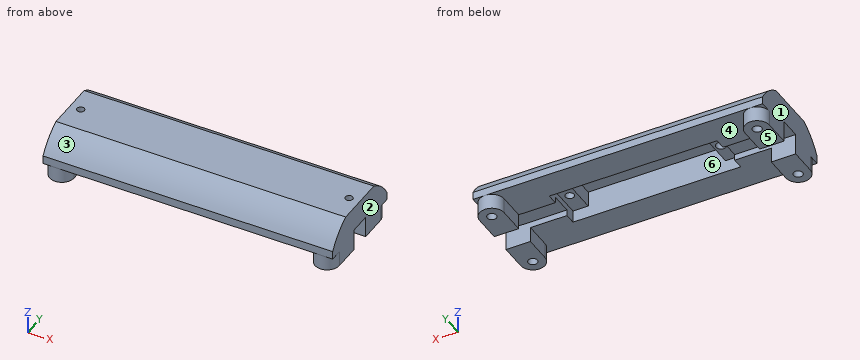
from build123d import *

# Parameters (mm, degrees)
SKETCH1_R             = 4
SKETCH1_R_2           = 1.5
BOSS_EXTRUDE1_DEPTH   = 5
BOSS_EXTRUDE1_2_DEPTH = 5
BOSS_EXTRUDE1_3_DEPTH = 5
BOSS_EXTRUDE1_4_DEPTH = 5
SKETCH2_W             = 95
SKETCH2_H             = 32.5
BOSS_EXTRUDE2_DEPTH   = 10
SKETCH3_W             = 45
SKETCH3_H             = 14.2
CUT_EXTRUDE1_DEPTH    = 9
SKETCH4_W             = 5
SKETCH4_H             = 14.2
SKETCH4_W_2           = 45
CUT_EXTRUDE2_DEPTH    = 4
SKETCH5_R             = 1.4
SKETCH5_R_2           = 1.6
CUT_EXTRUDE3_DEPTH    = 5
BOSS_EXTRUDE3_DEPTH   = 5
CUT_EXTRUDE5_DEPTH    = 96
SKETCH9_W             = 7
SKETCH9_H             = 7
CUT_EXTRUDE6_DEPTH    = 96
SKETCH10_R            = 1.2
CUT_EXTRUDE7_DEPTH    = 16


with BuildPart() as part:
    # Sketch1 → Boss-Extrude1 (new body)
    with BuildSketch(Plane.XY):
        with Locations((-43.5, -12.25)):
            Circle(SKETCH1_R)
        with Locations((-43.5, -12.25)):
            Circle(SKETCH1_R_2, mode=Mode.SUBTRACT)
    extrude(amount=BOSS_EXTRUDE1_DEPTH)



with BuildPart() as body_2:
    # Sketch1 → Boss-Extrude1 2 (new body)
    with BuildSketch(Plane.XY):
        with Locations((-43.5, 12.25)):
            Circle(SKETCH1_R)
        with Locations((-43.5, 12.25)):
            Circle(SKETCH1_R_2, mode=Mode.SUBTRACT)
    extrude(amount=BOSS_EXTRUDE1_2_DEPTH)


with BuildPart() as body_3:
    # Sketch1 → Boss-Extrude1 3 (new body)
    with BuildSketch(Plane.XY):
        with Locations((43.5, -12.25)):
            Circle(SKETCH1_R)
        with Locations((43.5, -12.25)):
            Circle(SKETCH1_R_2, mode=Mode.SUBTRACT)
    extrude(amount=BOSS_EXTRUDE1_3_DEPTH)


with BuildPart() as body_4:
    # Sketch1 → Boss-Extrude1 4 (new body)
    with BuildSketch(Plane.XY):
        with Locations((43.5, 12.25)):
            Circle(SKETCH1_R)
        with Locations((43.5, 12.25)):
            Circle(SKETCH1_R_2, mode=Mode.SUBTRACT)
    extrude(amount=BOSS_EXTRUDE1_4_DEPTH)


with BuildPart() as part_1:
    add(part.part)

    add(body_2.part)  # Boss-Extrude2 merges body 2

    add(body_3.part)  # Boss-Extrude2 merges body 3

    add(body_4.part)  # Boss-Extrude2 merges body 4
    # Sketch2 → Boss-Extrude2 (add)
    with BuildSketch(Plane.XY.offset(5)):
        Rectangle(SKETCH2_W, SKETCH2_H)
    extrude(amount=BOSS_EXTRUDE2_DEPTH)

    # Sketch3 → Cut-Extrude1 (cut)
    with BuildSketch(Plane(origin=(0, 0, 5), x_dir=(-1, 0, 0), z_dir=(0, 0, -1))):
        Rectangle(SKETCH3_W, SKETCH3_H)
    extrude(amount=-CUT_EXTRUDE1_DEPTH, mode=Mode.SUBTRACT)

    # Sketch4 → Cut-Extrude2 (cut)
    with BuildSketch(Plane(origin=(0, 0, 5), x_dir=(-1, 0, 0), z_dir=(0, 0, -1))):
        with Locations((-25, 0)):
            Rectangle(SKETCH4_W, SKETCH4_H)
        Rectangle(SKETCH4_W_2, SKETCH4_H)
        with Locations((25, 0)):
            Rectangle(SKETCH4_W, SKETCH4_H)
    extrude(amount=-CUT_EXTRUDE2_DEPTH, mode=Mode.SUBTRACT)

    # Sketch5 → Cut-Extrude3 (cut)
    with BuildSketch(Plane(origin=(0, 0, 9), x_dir=(-1, 0, 0), z_dir=(0, 0, -1))):
        with Locations((-24.8, -0.2)):
            Circle(SKETCH5_R)
        with Locations((24.8, -0.2)):
            Circle(SKETCH5_R_2)
    extrude(amount=-CUT_EXTRUDE3_DEPTH, mode=Mode.SUBTRACT)

    # Sketch6 → Boss-Extrude3 (add)
    with BuildSketch(Plane(origin=(0, 0, 5), x_dir=(-1, 0, 0), z_dir=(0, 0, -1))):
        with BuildLine():
            ThreePointArc((47.5, 12.25), (43.5, 8.25), (39.5, 12.25))
            Line((39.5, 12.25), (39.5, -12.25))
            ThreePointArc((39.5, -12.25), (43.5, -8.25), (47.5, -12.25))
            Line((47.5, -12.25), (47.5, 12.25))
        make_face()
        with BuildLine():
            ThreePointArc((-39.5, 12.25), (-43.5, 8.25), (-47.5, 12.25))
            Line((-47.5, 12.25), (-47.5, -12.25))
            ThreePointArc((-47.5, -12.25), (-43.5, -8.25), (-39.5, -12.25))
            Line((-39.5, -12.25), (-39.5, 12.25))
        make_face()
    extrude(amount=BOSS_EXTRUDE3_DEPTH)

    # Sketch8 → Cut-Extrude5 (cut, through all)
    with BuildSketch(Plane(origin=(47.5, 0, 0), x_dir=(0, 0, -1), z_dir=(1, 0, 0))):
        with BuildLine():
            ThreePointArc((-15, 8.377014021), (-11.841659381, 12.867099577), (-7.518238456, 16.25))
            Line((-7.518238456, 16.25), (-15, 16.25))
            Line((-15, 16.25), (-15, 8.377014021))
        make_face()
        with BuildLine():
            Line((-15, -16.25), (-7.688934819, -16.25))
            ThreePointArc((-7.688934819, -16.25), (-11.909309532, -12.893789895), (-15, -8.475267356))
            Line((-15, -8.475267356), (-15, -16.25))
        make_face()
    extrude(amount=-CUT_EXTRUDE5_DEPTH, mode=Mode.SUBTRACT)

    # Sketch9 → Cut-Extrude6 (cut, through all)
    with BuildSketch(Plane.ZY.offset(47.5)):
        with Locations((3.5, 0)):
            Rectangle(SKETCH9_W, SKETCH9_H)
    extrude(amount=-CUT_EXTRUDE6_DEPTH, mode=Mode.SUBTRACT)

    # Sketch10 → Cut-Extrude7 (cut, through all)
    with BuildSketch(Plane.XY.offset(15)):
        with Locations((-44, -0.049126667)):
            Circle(SKETCH10_R)
        with Locations((44, -0.049126667)):
            Circle(SKETCH10_R)
    extrude(amount=-CUT_EXTRUDE7_DEPTH, mode=Mode.SUBTRACT)


solid = part_1.part
Can you work these out from the model? Positions are in its coordinate system, mm. Face numbers are marked on the shaded views. A direction names the side the tool comes from. Coordinates: 2 decimals unless noted, no trailing zeros. Order: outer loops, then holes, each group sorted by start corner. A loop starts at its lowest first (then second) coordinate and runs counter-clockwise, first axis right, second up. Notation, with made-up numbers: M -26.5,5 L -2.5,5 A25 cw -2.5,28 Z; hole C 60,84 d11. An arc over 180 degrees is marked long. Write item = value, one per line.
(1) Suppose I cut it at A-A on z = 10.75. Please give me the cut outline in (x, y).
Results are:
outline = M -47.5,-14.02 L 47.5,-14.02 L 47.5,13.93 L -47.5,13.93 Z; hole C -44,-0.05 d2.4; hole C -24.8,-0.2 d3.2; hole M -22.5,-7.1 L 22.5,-7.1 L 22.5,7.1 L -22.5,7.1 Z; hole C 24.8,-0.2 d2.8; hole C 44,-0.05 d2.4
(2) I need wall thicknesses on line 1 along Y through (x, z) = (43.5, 1.6); line 2 along X through (y, z) = (0.5, 11.5); line 3 along X through (y, z) = (6, 7). Which ranges of each line are inside material? Lowest first, please. Write a range as [from, to].
Results are:
line_1 = [-16.25, -13.75], [-10.75, -3.5], [3.5, 10.75], [13.75, 16.25]
line_2 = [-47.5, -45.07], [-42.93, -26.24], [-23.36, -22.5], [22.5, 23.59], [26.01, 42.93], [45.07, 47.5]
line_3 = [-47.5, -27.5], [27.5, 47.5]
(3) Suppose I cut it at C-C on x = -11. Please give me the cut outline in (y, z), plus the area to 3 significant figures.
Results are:
outline = M -16.25,5 L -7.1,5 L -7.1,14 L 7.1,14 L 7.1,5 L 16.25,5 L 16.25,7.52 A18.75 ccw 8.38,15 L -8.48,15 A18.75 ccw -16.25,7.69 Z
area = 151 mm2
(4) If we mould it in two halves opening along X, with no side actions, what happens to the marked faces 1, 2, 3 and 4? For each: pulls with the +X half, pulls with the -X half, needs draft (parallel to the pull), parting line crosses it, or undercut.
Results are:
face_1 = pulls with the -X half
face_2 = pulls with the +X half
face_3 = needs draft
face_4 = undercut
(5) For pin 1 Ø4 at (x, y) = (-12.5, -0.5) entering from -Z; pin 2 Ø5 at (x, y) = (-43.5, 12.25) entering from +Z; pin 3 Ø10 at (x, y) = (7.5, -10) entering from -Z; pin 4 Ø2 at (x, z) = (-36.5, 3) entering from +Y, each with a flat end and sliding along its axis, tell me the tip position at first contact or that it passes through.
Results are:
pin_1 = 14
pin_2 = 14.24
pin_3 = 5
pin_4 = through
(6) Suppose I cut it at D-D on x = -24.8. Please give me the cut outline in (y, z).
Results are:
outline = M -16.25,5 L -7.1,5 L -7.1,9 L -1.8,9 L -1.8,14 L 1.4,14 L 1.4,9 L 7.1,9 L 7.1,5 L 16.25,5 L 16.25,7.52 A18.75 ccw 8.38,15 L -8.48,15 A18.75 ccw -16.25,7.69 Z
(7) For the marked faces 5 and 6, which set-ups out of +Z, -Z, +X, -X, +Y, -Y let a thin tool reach every point of the face, with its end or its side?
Results are:
face_5 = -Z, +X, -X, +Y, -Y
face_6 = -Z
(8) Suppose I cut it at B-B on y = 5. Please give me the cut outline in (x, z).
Results are:
outline = M -47.5,0 L -39.5,0 L -39.5,5 L -27.5,5 L -27.5,9 L -22.5,9 L -22.5,14 L 22.5,14 L 22.5,9 L 27.5,9 L 27.5,5 L 39.5,5 L 39.5,0 L 47.5,0 L 47.5,15 L -47.5,15 Z
